```python
from build123d import *

# Parameters (mm, degrees)
SKETCH_1_R               = 10
EXTRUDE_2_DEPTH          = 36.5
CUT_EXTRUDE_1_DEPTH      = 40.143965052
CUT_EXTRUDE_1_DEPTH_BACK = 40.143965052
SKETCH_3_W               = 8
SKETCH_3_H               = 28
CUT_EXTRUDE_2_DEPTH      = 40.143965052
CUT_EXTRUDE_2_DEPTH_BACK = 40.143965052
SKETCH_4_W               = 2
SKETCH_4_H               = 36.5
CUT_EXTRUDE_4_DEPTH      = 39.681390875
CUT_EXTRUDE_4_DEPTH_BACK = 39.681390875
SKETCH_6_R               = 2.25
SKETCH_7_R               = 2.85
CUT_EXTRUDE_5_DEPTH      = 3.8
SKETCH_8_R               = 0.8
CUT_EXTRUDE_6_DEPTH      = 42.088319508


with BuildPart() as part:
    # 草图1 → 凸台-拉伸2 (new body)
    with BuildSketch(Plane.XY):
        Circle(SKETCH_1_R)
    extrude(amount=EXTRUDE_2_DEPTH)

    # 草图3 → 切除-拉伸1 (cut, two sides: drawn at the far end of the back side and taken through both)
    with BuildSketch(Plane(origin=(0, 0, 0), x_dir=(1, 0, 0), z_dir=(0, 1, 0)).offset(-CUT_EXTRUDE_1_DEPTH_BACK)):
        with Locations((0, -22.5)):
            Rectangle(SKETCH_3_W, SKETCH_3_H)
    extrude(amount=CUT_EXTRUDE_1_DEPTH + CUT_EXTRUDE_1_DEPTH_BACK, mode=Mode.SUBTRACT)

    # 草图4 → 切除-拉伸2 (cut, two sides: drawn at the far end of the back side and taken through both)
    with BuildSketch(Plane(origin=(0, 0, 0), x_dir=(1, 0, 0), z_dir=(0, 1, 0)).offset(-CUT_EXTRUDE_2_DEPTH_BACK)):
        with Locations((-9, -18.25)):
            Rectangle(SKETCH_4_W, SKETCH_4_H)
        with Locations((9, -18.25)):
            Rectangle(SKETCH_4_W, SKETCH_4_H)
    extrude(amount=CUT_EXTRUDE_2_DEPTH + CUT_EXTRUDE_2_DEPTH_BACK, mode=Mode.SUBTRACT)

    # 草图6 → 切除-拉伸4 (cut, two sides: drawn at the far end of the back side and taken through both)
    with BuildSketch(Plane(origin=(0, 0, 0), x_dir=(0, 0, -1), z_dir=(1, 0, 0)).offset(-CUT_EXTRUDE_4_DEPTH_BACK)):
        with Locations((-28, 0)):
            Circle(SKETCH_6_R)
    extrude(amount=CUT_EXTRUDE_4_DEPTH + CUT_EXTRUDE_4_DEPTH_BACK, mode=Mode.SUBTRACT)

    # 草图7 → 切除-拉伸5 (cut)
    with BuildSketch(Plane(origin=(0, 0, 0), x_dir=(-1, 0, 0), z_dir=(0, 0, -1))):
        Circle(SKETCH_7_R)
    extrude(amount=-CUT_EXTRUDE_5_DEPTH, mode=Mode.SUBTRACT)

    # 草图8 → 切除-拉伸6 (cut, through all)
    with BuildSketch(Plane.ZY.offset(8)):
        with Locations((1.7, 0)):
            Circle(SKETCH_8_R)
    extrude(amount=-CUT_EXTRUDE_6_DEPTH, mode=Mode.SUBTRACT)


solid = part.part
```
The listing builds one solid part. Answer for the finished solid, in the listing's coordinates (mm). A direction names the side the tool comes from. Give positions to 0.01 mm unless a question says otherwise; leave off trailing zeros. Order: outer loops, then holes, each group sorted by start corner. A loop starts at its lowest first (then second) coordinate and runs counter-clockwise, first axis right, second up.
Item 1: The part is cut by section D-D, the plane x = 0. Give the vertices of the cut face in (y, z).
From the geometry:
outline: (-10, 0) - (-2.85, 0) - (-2.85, 3.8) - (2.85, 3.8) - (2.85, 0) - (10, 0) - (10, 8.5) - (-10, 8.5) - close
Item 2: For a pull along Z with two mould halves and no side action, classify faces 1 (the face through (-6.028, 0.676, 25.854)), 2 (the face through (4, 0, 23)), 3 (the face through (-5.405, 0.24, 2.463)), 4 (the face through (6, 0, 36.5)) as pulls with the +Z half, pulls with the -Z half, needs draft (parallel to the pull), parting line crosses it, or undercut.
From the geometry:
face 1: undercut
face 2: needs draft
face 3: undercut
face 4: pulls with the +Z half
Item 3: The part is cut by section A-A, the plane y = 0. Give the vertices of the cut face in (x, z), and give its area (3 significant figures).
From the geometry:
outline: (-8, 0) - (-2.85, 0) - (-2.85, 0.9) - (-8, 0.9) - close; (-8, 2.5) - (-2.85, 2.5) - (-2.85, 3.8) - (2.85, 3.8) - (2.85, 2.5) - (8, 2.5) - (8, 25.75) - (4, 25.75) - (4, 8.5) - (-4, 8.5) - (-4, 25.75) - (-8, 25.75) - close; (-8, 30.25) - (-4, 30.25) - (-4, 36.5) - (-8, 36.5) - close; (2.85, 0) - (8, 0) - (8, 0.9) - (2.85, 0.9) - close; (4, 30.25) - (8, 30.25) - (8, 36.5) - (4, 36.5) - close
area: 286 mm2
Item 4: Given pin 1 Ø5 at (x, z) = (6, 20) entering from -Y; pin 2 Ø5 at (x, y) = (0, 0) entering from -Z; pin 3 Ø2.5 at (x, y) = (-1.5, -0.5) entering from +Z, each flat-ended and moving along its own axis, determine where each tip first touches the part or whether it passes through.
From the geometry:
pin 1: stops at y = -9.17
pin 2: stops at z = 3.8
pin 3: stops at z = 8.5
Item 5: Which of the six approach directions +Z, -Z, +X, -X, +Y, -Y give full straight-line access (tool end or side, diameter ignored) to faces 5 (the face through (-4, 0, 23)), 6 (the face through (0, 0, 3.8)), 7 (the face through (-6, -8, 14))?
From the geometry:
face 5: +Z, +Y, -Y
face 6: -Z
face 7: +Z, -Z, -Y
Item 6: The part is cut by section B-B, the plane z = 10. Give the vertices of the cut face in (x, y), and give its area (3 significant figures).
From the geometry:
outline: (-8, -6) arc R10 ccw to (-4, -9.17) - (-4, 9.17) arc R10 ccw to (-8, 6) - close; (4, -9.17) arc R10 ccw to (8, -6) - (8, 6) arc R10 ccw to (4, 9.17) - close
area: 126 mm2
Item 7: Find the intervals of material crossed by probe 1 along Z at (x, y) = (4.15, 0); probe 2 along X at (y, z) = (3.5, 17.5); probe 3 along Y at (x, z) = (0, 1.4), in increasing order.
From the geometry:
probe 1: z = 0 to 0.9, 2.5 to 25.75, 30.25 to 36.5
probe 2: x = -8 to -4, 4 to 8
probe 3: y = -10 to -2.85, 2.85 to 10
Item 8: The part is cut by section C-C, the plane z = 28. Give the vertices of the cut face in (x, y).
From the geometry:
outline: (-8, -6) arc R10 ccw to (-4, -9.17) - (-4, -2.25) - (-8, -2.25) - close; (-8, 2.25) - (-4, 2.25) - (-4, 9.17) arc R10 ccw to (-8, 6) - close; (4, -9.17) arc R10 ccw to (8, -6) - (8, -2.25) - (4, -2.25) - close; (4, 2.25) - (8, 2.25) - (8, 6) arc R10 ccw to (4, 9.17) - close
